CAD build for the part. Positions are in the model's coordinates, mm. A direction names the side the tool comes from. Give positions to 0.01 mm unless a question says otherwise; leave off trailing zeros. Order: outer loops, then holes, each group sorted by start corner. A loop starts at its lowest first (then second) coordinate and runs counter-clockwise, first axis right, second up.
Item 1: Band-saw the part on D-D on x = 0. Give the cut face in (y, z).
Item 2: Band-saw the part on C-C on z = 4. Give the cut face in (x, y), plus the area to 3 significant figures.
Item 3: Flat gauge pins, fed straight in: P1, Ø2.5, axis at x = -1, y = 4.5, coming from the +Z side; P2, Ø1, axis at x = 0.5, z = 9.5, coming from the -Y side; P3, Ø2, axis at x = 3, z = 10, coming from the +Y side; P4, Ø3, axis at x = 3, z = 9, coming from the +Y side. Where does each tip first touch, or does it go through?
Item 4: Band-saw the part on A-A on y = -12. Give the cut face in (x, z), plus the area to 3 significant figures.
Item 5: Which spindle directions (+Z, -Z, +X, -X, +Y, -Y) get a long thin tool onto all of the face, cutting with end or side? Do faces 1 (the flat face through (-0.21, 0.1, 3.05)), 2 (the flat face through (0, 13, 8)), 3 (the cylindrical face through (-1.327, -15.168, 5.916)), 4 (the cylindrical face through (8.5, 11.7, 3.4)). Say none if no direction does.
Item 6: Wall check: L1, parallel to X at y = -1.5, z = 1.75; L2, parallel to X at y = -12, z = 3; L3, parallel to Y at x = 13.5, z = 5. Give the ranges that are in metal, low to high.
Item 7: Two-plate mould, pull along Y, no slides. Class faces 5 (the flat face through (15, -3, 5)), 6 (the cylindrical face through (0, -9, 6)), 7 (the flat face through (0, 15.5, 4)): released by +Y, released by -Y, zero draft, split by the parting line, or undercut.
Item 8: Band-saw the part on B-B on x = 7.5. Give the cut face in (y, z), plus the area to 3 significant figures.
```python
from build123d import *

# Parameters (mm, degrees)
SKETCH003_R     = 8.5
PAD001_DEPTH    = 3
SKETCH004_R     = 6.5
POCKET002_DEPTH = 3.001
PAD_DEPTH       = 12
POCKET_DEPTH    = 30.001
SKETCH002_W     = 5.95
SKETCH002_H     = 4
POCKET001_DEPTH = 30.001


with BuildPart() as pocket002:
    # Sketch003 → Pad001 (new body)
    with BuildSketch(Plane.YZ.offset(10)):
        with Locations((4, 7)):
            Circle(SKETCH003_R)
    extrude(amount=-PAD001_DEPTH)

    # Sketch004 → Pocket002 (cut, through all)
    with BuildSketch(Plane.YZ.offset(10)):
        with Locations((4, 7)):
            Circle(SKETCH004_R)
    extrude(amount=-POCKET002_DEPTH, mode=Mode.SUBTRACT)


with BuildPart() as part_mirroring:
    # Part__Mirroring: instance of Pocket002
    add(pocket002.part.mirror(Plane(origin=(0, 0, 0), x_dir=(0, -1, 0), z_dir=(1, 0, 0))))


with BuildPart() as cut001:
    # Sketch → Pad (new body)
    with BuildSketch(Plane.XY):
        with BuildLine():
            Line((-15, 15.5), (15, 15.5))
            Line((15, 15.5), (15, -15.5))
            Line((1.848981, -15.5), (15, -15.5))
            ThreePointArc((1.543183, -14.572662), (1.323663, -15.159139), (1.848981, -15.5))
            ThreePointArc((1.543183, -14.572662), (0, -9), (-1.543183, -14.572662))
            ThreePointArc((-1.848981, -15.5), (-1.323663, -15.159139), (-1.543183, -14.572662))
            Line((-15, -15.5), (-1.848981, -15.5))
            Line((-15, -15.5), (-15, 15.5))
        make_face()
    extrude(amount=PAD_DEPTH)

    # Sketch001 → Pocket (cut, through all)
    with BuildSketch(Plane(origin=(-15, 0, 0), x_dir=(0, -1, 0), z_dir=(-1, 0, 0))):
        Polygon((1.55, 4.701115), (1.55, 9.298885), (1.55, 12), (-9.55, 12), (-9.55, 9.298885), (-9.55, 4.701115), (-6.298885, 1.45), (-1.701115, 1.45), align=None)
    extrude(amount=-POCKET_DEPTH, mode=Mode.SUBTRACT)

    # Sketch002 → Pocket001 (cut, through all)
    with BuildSketch(Plane(origin=(-15, 0, 0), x_dir=(0, -1, 0), z_dir=(-1, 0, 0))):
        with Locations((-12.525, 10)):
            Rectangle(SKETCH002_W, SKETCH002_H)
    extrude(amount=-POCKET001_DEPTH, mode=Mode.SUBTRACT)

    # Cut: cut Part__Mirroring
    add(part_mirroring.part, mode=Mode.SUBTRACT)

    # Cut001: cut Pocket002
    add(pocket002.part, mode=Mode.SUBTRACT)


solid = cut001.part
```
The answers:
1. outline: (-9, 0) - (15.5, 0) - (15.5, 8) - (9.55, 8) - (9.55, 4.7) - (6.3, 1.45) - (1.7, 1.45) - (-1.55, 4.7) - (-1.55, 12) - (-9, 12) - close
2. outline: (-15, -15.5) - (-1.85, -15.5) arc R0.5 ccw to (-1.54, -14.57) arc R3 cw (long way) to (1.54, -14.57) arc R0.5 ccw to (1.85, -15.5) - (15, -15.5) - (15, -0.85) - (-15, -0.85) - close; (-15, 8.85) - (15, 8.85) - (15, 15.5) - (-15, 15.5) - close; hole (-10, -3.95) - (-7, -3.95) - (-7, -1.77) - (-10, -1.77) - close; hole (-10, 9.77) - (-7, 9.77) - (-7, 11.95) - (-10, 11.95) - close; hole (7, -3.95) - (10, -3.95) - (10, -1.77) - (7, -1.77) - close; hole (7, 9.77) - (10, 9.77) - (10, 11.95) - (7, 11.95) - close
2. area: 583 mm2
3. P1: stops at z = 1.45
3. P2: stops at y = -9.17
3. P3: stops at y = -1.55
3. P4: stops at y = 15.5
4. outline: (-15, 0) - (-3, 0) - (-3, 12) - (-15, 12) - close; (3, 0) - (15, 0) - (15, 12) - (3, 12) - close
4. area: 288 mm2
5. face 1: +Z, +X, -X
5. face 2: +Z, +X, -X, +Y
5. face 3: +Z, -Z
5. face 4: none
6. L1: x = -15 to -10, -7 to 7, 10 to 15
6. L2: x = -15 to -3, 3 to 15
6. L3: y = -15.5 to -1.55, 9.55 to 15.5
7. face 5: zero draft
7. face 6: undercut
7. face 7: released by +Y
8. outline: (-15.5, 0) - (-0.82, 0) arc R8.5 cw to (-2.87, 12) - (-15.5, 12) - close; (-1.55, 4.7) - (-1.55, 10.38) arc R6.5 ccw (long way) to (10.42, 8) - (9.55, 8) - (9.55, 4.7) - (6.3, 1.45) - (1.7, 1.45) - close; (8.82, 0) - (15.5, 0) - (15.5, 8) - (12.44, 8) arc R8.5 cw to start
8. area: 192 mm2
